```python
from build123d import *

# Parameters (mm, degrees)
SKETCH1_R               = 22.5
BOSS_EXTRUDE1_DEPTH     = 4
SKETCH2_R               = 17.5
BOSS_EXTRUDE2_DEPTH     = 24
SKETCH3_R               = 16
CUT_EXTRUDE1_DEPTH      = 20
SKETCH4_R               = 3
BOSS_EXTRUDE3_DEPTH     = 6
SKETCH6_R               = 1.5
CUT_EXTRUDE3_DEPTH      = 8
SKETCH7_R               = 1.5
CUT_EXTRUDE4_DEPTH      = 10
CUT_EXTRUDE5_REACH      = 53.79
CUT_EXTRUDE5_END_RADIUS = 16
SKETCH10_R              = 6
FILLET1_R               = 2.5
FILLET2_R               = 1


with BuildPart() as part:
    # Sketch1 → Boss-Extrude1 (new body)
    with BuildSketch(Plane(origin=(0, 0, 0), x_dir=(1, 0, 0), z_dir=(0, 1, 0))):
        with Locations(Location((0, 0, 0), (0, 0, 270))):
            Circle(SKETCH1_R)
    extrude(amount=BOSS_EXTRUDE1_DEPTH)

    # Sketch2 → Boss-Extrude2 (add)
    with BuildSketch(Plane(origin=(0, 0, 0), x_dir=(1, 0, 0), z_dir=(0, 1, 0))):
        with Locations(Location((0, 0, 0), (0, 0, 270))):
            Circle(SKETCH2_R)
    extrude(amount=-BOSS_EXTRUDE2_DEPTH)

    # Sketch3 → Cut-Extrude1 (cut)
    with BuildSketch(Plane(origin=(0, 4, 0), x_dir=(1, 0, 0), z_dir=(0, 1, 0))):
        with Locations(Location((0, 0, 0), (0, 0, 270))):
            Circle(SKETCH3_R)
    extrude(amount=-CUT_EXTRUDE1_DEPTH, mode=Mode.SUBTRACT)

    # Sketch4 → Boss-Extrude3 (add)
    with BuildSketch(Plane(origin=(0, -16, 0), x_dir=(1, 0, 0), z_dir=(0, 1, 0))):
        with Locations(Location((-8, 8, 0), (0, 0, 270))):
            Circle(SKETCH4_R)
        with Locations(Location((8, 8, 0), (0, 0, 270))):
            Circle(SKETCH4_R)
        with Locations(Location((-8, -8, 0), (0, 0, 270))):
            Circle(SKETCH4_R)
        with Locations(Location((8, -8, 0), (0, 0, 270))):
            Circle(SKETCH4_R)
    extrude(amount=BOSS_EXTRUDE3_DEPTH)

    # Sketch6 → Cut-Extrude3 (cut)
    with BuildSketch(Plane(origin=(0, -10, 0), x_dir=(1, 0, 0), z_dir=(0, 1, 0))):
        with Locations(Location((-8, 8, 0), (0, 0, 270))):
            Circle(SKETCH6_R)
        with Locations(Location((8, 8, 0), (0, 0, 270))):
            Circle(SKETCH6_R)
        with Locations(Location((8, -8, 0), (0, 0, 270))):
            Circle(SKETCH6_R)
        with Locations(Location((-8, -8, 0), (0, 0, 270))):
            Circle(SKETCH6_R)
    extrude(amount=-CUT_EXTRUDE3_DEPTH, mode=Mode.SUBTRACT)

    # Sketch7 → Cut-Extrude4 (cut)
    with BuildSketch(Plane(origin=(0, 4, 0), x_dir=(1, 0, 0), z_dir=(0, 1, 0))):
        with Locations(Location((-0.875515832, 19.230079876, 0), (0, 0, 270))):
            Circle(SKETCH7_R)
        with Locations(Location((17.091495605, -8.856820986, 0), (0, 0, 270))):
            Circle(SKETCH7_R)
        with Locations(Location((-16.215979773, -10.37325889, 0), (0, 0, 270))):
            Circle(SKETCH7_R)
    extrude(amount=-CUT_EXTRUDE4_DEPTH, mode=Mode.SUBTRACT)

    # Cut-Extrude5: up to this cylinder (the profile starts outside it)
    cut_extrude5_end = Plane(origin=(0, -10, 0), z_dir=(0, 1, 0)) * Cylinder(CUT_EXTRUDE5_END_RADIUS, 140.58, mode=Mode.PRIVATE)
    # Sketch10 → Cut-Extrude5 (cut, up to the surface)
    with BuildSketch(Plane.XY.offset(17.5), mode=Mode.PRIVATE) as cut_extrude5_sk1:
        with Locations(Location((0, -10, 0), (0, 0, 90))):
            Circle(SKETCH10_R)
    cut_extrude5_tool1 = extrude(cut_extrude5_sk1.sketch, amount=-CUT_EXTRUDE5_REACH, mode=Mode.PRIVATE) - cut_extrude5_end
    add(cut_extrude5_tool1.solids().sort_by_distance((0, -10, 17.5))[0], mode=Mode.SUBTRACT)

    # Fillet1
    fillet1_edges = [part.edges().sort_by_distance(p)[0] for p in [
        (0, -24, -17.5),
    ]]
    fillet(fillet1_edges, radius=FILLET1_R)

    # Fillet2
    fillet2_edges = [part.edges().sort_by_distance(p)[0] for p in [
        (0, 0, -22.5),
    ]]
    fillet(fillet2_edges, radius=FILLET2_R)


solid = part.part
```
Check sheet for the modelled part. Datum: model origin and axes. Units: mm. A direction names the side the tool comes from. Round coordinates to 2 decimals unless told otherwise and drop trailing zeros. Order: outer loops, then holes, each group sorted by start corner. A loop starts at its lowest first (then second) coordinate and runs counter-clockwise, first axis right, second up. Notation, with made-up numbers: (73, -7) -> (100, -7) arc R16 cw to (100, 6) -> close; hole circle Ø2 at (44.25, 9). An arc over 180 degrees is marked (long way). One line per item, written item: value. Start each with the question number.
Q1. Cross-section at C-C (y = -20.5). Record the boundary of the cut face in (x, z), and give its area (3 significant figures).
Q2. Set-up check for faces 4 (the face through (3.65, -14.76, 16.18)), 5 (the face through (-17.4, 0, -3.3)), 6 (the face through (8, -18, 8)): record each of +Z, -Z, +X, -X, +Y, -Y from which the full face is reachable in a straight line by a thin tool's end or side.
Q3. Cross-section at B-B (z = 0). Record the boundary of the cut face in (x, y), and give its area (3 significant figures).
Q4. Gauge pin test, flat ends, axial feed: pin 1 Ø5 at (x, z) = (-0.88, -19.23) entering from -Y; pin 2 Ø3.5 at (x, z) = (7.5, -8.5) entering from +Y; pin 3 Ø1.8 at (x, z) = (17.09, 8.86) entering from +Y; pin 4 Ø4 at (x, y) = (-17, -12) entering from -Z. Record the tip position at first contact, or that the pin passes through.
Q5. Thickness scan on line 1 (X direction, y = -15.75, z = -8); line 2 (X direction, y = -15.25, z = -10); line 3 (Y direction, x = -8.5, z = 7.5). Record the ranges inside material, lowest first.
Q6. Cross-section at A-A (y = -11). Give the number of separate pieces and of enclosed holes in the cut face, and give its area (3 significant figures).
Q7. Mould release check, pull along Z, two halves, no side actions. Record for faces 1 (the face through (18.58, 2.03, 8.66)), 2 (the face through (0, -24, 0)), 3 (the face through (-10.648, -10.599, -13.887)): pulls with the +Z half, pulls with the -Z half, needs draft (parallel to the pull), parting line crosses it, or undercut.
Completed:
1. outline: circle Ø35 at (0, 0)
1. area: 962 mm²
2. face 4: +Z
2. face 5: -Y
2. face 6: +Y
3. outline: (-22.5, 1) arc R1 ccw to (-21.5, 0) -> (-17.5, 0) -> (-17.5, -21.5) arc R2.5 ccw to (-15, -24) -> (15, -24) arc R2.5 ccw to (17.5, -21.5) -> (17.5, 0) -> (21.5, 0) arc R1 ccw to (22.5, 1) -> (22.5, 4) -> (16, 4) -> (16, -16) -> (-16, -16) -> (-16, 4) -> (-22.5, 4) -> close
3. area: 377 mm²
4. pin 1: stops at y = -23.29
4. pin 2: stops at y = -10
4. pin 3: passes through
4. pin 4: stops at z = -9.01
5. line 1: x = -15.56 to -13.86, -11 to -9.5, -6.5 to -5, 5 to 6.5, 9.5 to 11, 13.86 to 15.56
5. line 2: x = -14.36 to -12.49, -10.24 to -5.76, 5.76 to 10.24, 12.49 to 14.36
5. line 3: y = -24 to -18
6. separate pieces: 5
6. enclosed holes: 4
6. area: 225 mm²
7. face 1: undercut
7. face 2: needs draft
7. face 3: parting line crosses it
